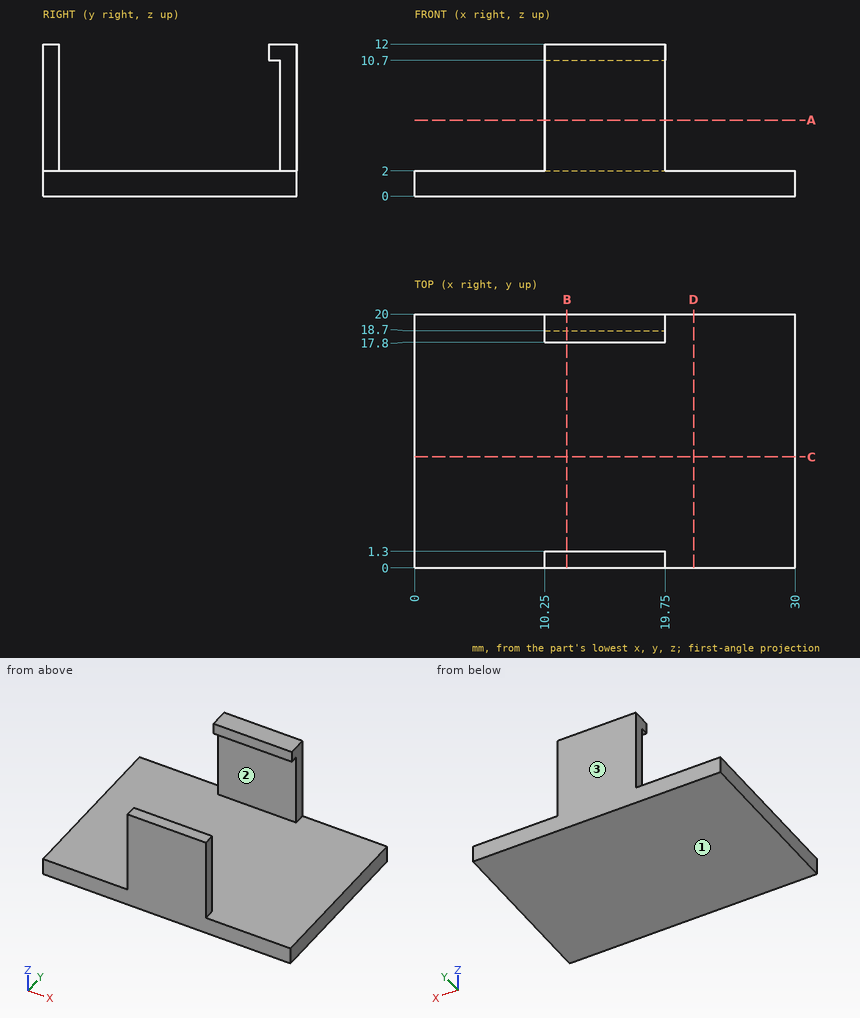
Geometry: see drawing. Coordinates: mm, zero at the bounding-box minimum. Coordinates: 2 decimals unless noted, no trailing zeros. Order: outer loops, then holes, each group sorted by start corner. A loop starts at its lowest first (then second) coordinate and runs counter-clockwise, first axis right, second up. Notation, with made-up numbers: M 30.5,57.5 L 36.5,57.5 A19 cw 36.5,78.5 Z; hole C -3,-6 d8. An arc over 180 degrees is marked long. Write each question's results on one line, items separated by ' | '. Start each with the question number.
1) Line query: line 1 (Y direction, x = 16.5, z = 11); line 2 (Y direction, x = 15, z = 9.75); line 3 (Z direction, x = 12.75, y = 17). Output: solid intervals per line, ascending. Write a range as from..to.
2) Section query B-B (x = 12). Return the cut outline in (y, z).
3) Section query A-A (z = 6). Return the cut outline in (x, y).
4) Contact query for flat-ended pins moving along their axis: pin 1 Ø2.5 at (y, z) = (19, 8.5) entering from -X; pin 2 Ø2 at (x, y) = (21.5, 10.5) entering from +Z; pin 3 Ø0.7 at (y, z) = (0.5, 5.5) entering from +X. Output: stop coordinate, or through.
5) Draft query along Z for the marked faces 1, 2 and 3. Return one class per face: released by +Z, released by -Z, zero draft, split by the parting line, or undercut.
6) Section query D-D (x = 22). Return the cut outline in (y, z), plus the area to 3 significant figures.
7) Section query C-C (y = 8.75). Return the cut outline in (x, z).
Answers:
1) line 1: y = 0..1.3, 17.8..20 | line 2: y = 0..1.3, 18.7..20 | line 3: z = 0..2
2) outline: M 0,0 L 20,0 L 20,12 L 17.8,12 L 17.8,10.7 L 18.7,10.7 L 18.7,2 L 1.3,2 L 1.3,12 L 0,12 Z
3) outline: M 10.25,0 L 19.75,0 L 19.75,1.3 L 10.25,1.3 Z; M 10.25,18.7 L 19.75,18.7 L 19.75,20 L 10.25,20 Z
4) pin 1: stops at x = 10.25 | pin 2: stops at z = 2 | pin 3: stops at x = 19.75
5) face 1: released by -Z | face 2: undercut | face 3: zero draft
6) outline: M 0,0 L 20,0 L 20,2 L 0,2 Z | area: 40.0 mm^2
7) outline: M 0,0 L 30,0 L 30,2 L 0,2 Z
